```python
from build123d import *

# Parameters (mm, degrees)
F0_W     = 160
F0_H     = 155
F0_R     = 1.75
F1_DEPTH = 1.5
F2_W     = 50.5
F2_H     = 27
F3_DEPTH = 1.5
F4_R     = 1.75
F5_DEPTH = 25
F6_R     = 3.5
F7_R     = 10


with BuildPart() as f1:
    # F0 (on Top) → F1 (new body)
    with BuildSketch(Plane.XY):
        Rectangle(F0_W, F0_H)
        with Locations((-74.75, -72)):
            Circle(F0_R, mode=Mode.SUBTRACT)
        with Locations((74.75, -72)):
            Circle(F0_R, mode=Mode.SUBTRACT)
        with Locations((-74.75, 37)):
            Circle(F0_R, mode=Mode.SUBTRACT)
        with Locations((74.75, 37)):
            Circle(F0_R, mode=Mode.SUBTRACT)
    extrude(amount=F1_DEPTH)

    # F2 (on Top) → F3 (join)
    with BuildSketch(Plane.XY):
        with Locations((54.75, -91)):
            Rectangle(F2_W, F2_H)
    extrude(amount=F3_DEPTH)

    # F4 (on face) → F5 (cut)
    with BuildSketch(Plane.XY.offset(1.5)):
        with Locations((76.75, -101)):
            Circle(F4_R)
        with Locations((32.75, -101)):
            Circle(F4_R)
        with Locations((32.75, -24)):
            Circle(F4_R)
        with Locations((76.75, -24)):
            Circle(F4_R)
    extrude(amount=-F5_DEPTH, mode=Mode.SUBTRACT)

    # F6
    f6_edges = [f1.edges().sort_by_distance(p)[0] for p in [
        (80, -104.5, 0.75),
        (29.5, -104.5, 0.75),
        (29.5, -77.5, 0.75),
        (-80, -77.5, 0.75),
    ]]
    fillet(f6_edges, radius=F6_R)

    # F7
    f7_edges = [f1.edges().sort_by_distance(p)[0] for p in [
        (80, 77.5, 0.75),
        (-80, 77.5, 0.75),
    ]]
    fillet(f7_edges, radius=F7_R)


solid = f1.part
```
Design review of the part built by this model. Coordinates are the model's own, in mm. Coordinates: 2 decimals unless noted, no trailing zeros. Loops run counter-clockwise (first coordinate to the right, second up) from the corner with the lowest first, then second, coordinate; pieces in that order, holes last.
Q1. To check wall thickness, follow line 1 (Y direction, x = 32.75, z = 1.2); line 2 (X direction, y = -72, z = 0.6); line 3 (X direction, y = -101, z = 1.15). State the ranges of each line that lie inside material, in increasing order.
Reported:
line 1: y = -104.49 to -102.75, -99.25 to -25.75, -22.25 to 77.5
line 2: x = -80 to -76.5, -73 to 73, 76.5 to 80
line 3: x = 29.5 to 31, 34.5 to 75, 78.5 to 80
Q2. We need section C-C on x = 19. State the section outline as (y, z) points, and give its area (4 significant figures).
Reported:
outline: (-77.5, 0) - (77.5, 0) - (77.5, 1.5) - (-77.5, 1.5) - close
area: 232.5 mm2
Q3. We need section B-B on y = -85. State the section outline as (x, z) points.
Reported:
outline: (29.5, 0) - (80, 0) - (80, 1.5) - (29.5, 1.5) - close
Q4. We need section A-A on z = 0.7. State how many separate pieces and enclosed holes the cut face has, and give its area (3 significant figures).
Reported:
separate pieces: 1
enclosed holes: 8
area: 26,000 mm2
Q5. For pin 1 (3 mm diameter, centred on x = 76.75, y = -101, fed in from +Z); pin 2 (10 mm diameter, centred on x = 55, y = -35, fed in from -Z), all flat-tipped, find the tip position at first contact; note any pin that passes through.
Reported:
pin 1: passes through
pin 2: stops at z = 0
